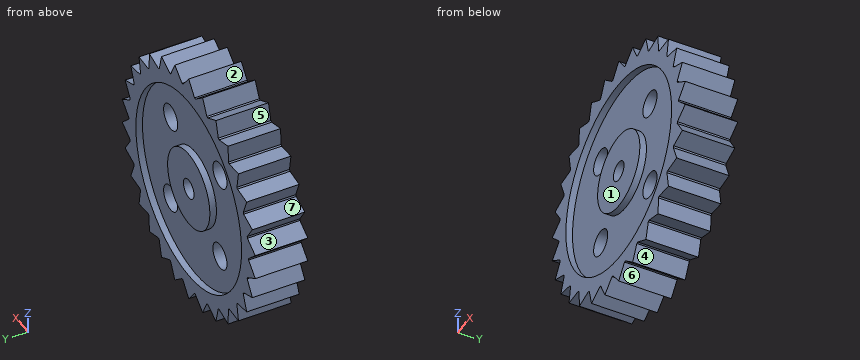
```python
from build123d import *

# Parameters (mm, degrees)
F0_R             = 13.49375
F1_DEPTH         = 3.175
F3_DEPTH         = 6.35
F3_COPIES_COUNT  = 30
F4_R             = 11.90625
F5_DEPTH         = 0.79375
F6_R             = 11.90625
F7_DEPTH         = 0.79375
F9_R             = 4.7625
F10_DEPTH        = 0.79375
F8_R             = 4.7625
F11_DEPTH        = 0.79375
F12_R            = 1.190625
F13_DEPTH        = 6.351
F14_R            = 1.5875
F15_DEPTH        = 5.55725
F15_COPIES_COUNT = 4


# Not quite as in the source:
# - a pattern or mirror of a feature is missing from the dataset's text; its kind, count and spacing are read off the source's solid


with BuildPart() as f1:
    # F0 (on Front) → F1 (new body, symmetric)
    with BuildSketch(Plane.XZ):
        Circle(F0_R)
    extrude(amount=F1_DEPTH, both=True)

    # F2 (on face) → F3 (join, through all)
    with BuildSketch(Plane.XZ.offset(3.175)):
        with BuildLine():
            Line((0, 15.08125), (-1.3182605719, 13.4292024382))
            ThreePointArc((-1.3182605719, 13.4292024382), (-0.6599199427, 13.4776034491), (0, 13.49375))
            Line((0, 13.49375), (0, 15.08125))
        make_face()
        with BuildLine():
            Line((1.2989129689, 13.4310876016), (0, 15.08125))
            Line((0, 15.08125), (0, 13.49375))
            ThreePointArc((0, 13.49375), (0.650211788, 13.4780752963), (1.2989129689, 13.4310876016))
        make_face()
    f3 = extrude(amount=-F3_DEPTH)

    # F3_copies: F3 ×30 about axis
    f3_copies_axis = Axis((0, 0, 0), (0, 1, 0))
    for i in range(1, F3_COPIES_COUNT):
        add(f3.rotate(f3_copies_axis, i * 360 / F3_COPIES_COUNT))

    # F4 (on face) → F5 (cut)
    with BuildSketch(Plane.XZ.offset(3.175)):
        Circle(F4_R)
    extrude(amount=-F5_DEPTH, mode=Mode.SUBTRACT)

    # F6 (on face) → F7 (cut)
    with BuildSketch(Plane(origin=(0, 3.175, 0), x_dir=(-1, 0, 0), z_dir=(0, 1, 0))):
        Circle(F6_R)
    extrude(amount=-F7_DEPTH, mode=Mode.SUBTRACT)

    # F9 (on face) → F10 (join)
    with BuildSketch(Plane(origin=(0, 2.38125, 0), x_dir=(-1, 0, 0), z_dir=(0, 1, 0))):
        Circle(F9_R)
    extrude(amount=F10_DEPTH)

    # F8 (on face) → F11 (join)
    with BuildSketch(Plane.XZ.offset(2.38125)):
        Circle(F8_R)
    extrude(amount=F11_DEPTH)

    # F12 (on face) → F13 (cut, through all)
    with BuildSketch(Plane.XZ.offset(3.175)):
        Circle(F12_R)
    extrude(amount=-F13_DEPTH, mode=Mode.SUBTRACT)

    # F14 (on face) → F15 (cut, through all)
    with BuildSketch(Plane.XZ.offset(2.38125)):
        with Locations((5.55625, -5.55625)):
            Circle(F14_R)
    f15 = extrude(amount=-F15_DEPTH, mode=Mode.SUBTRACT)

    # F15_copies: F15 ×4 about axis
    f15_copies_axis = Axis((0, 0, 0), (0, 1, 0))
    for i in range(1, F15_COPIES_COUNT):
        add(f15.rotate(f15_copies_axis, i * 360 / F15_COPIES_COUNT), mode=Mode.SUBTRACT)


solid = f1.part
```
Build history of the part. All positions in model axes, mm. Face numbers are marked on the shaded views. A direction names the side the tool comes from. Round coordinates to 2 decimals unless told otherwise and drop trailing zeros. Write each loop counter-clockwise with the first axis right and the second up, starting at its lowest first coordinate (ties: lowest second). Pieces come first, ordered by that corner, then holes.
1) Mould opens along X. For the marked faces 1, 2, 3 and 4 say: +X half, -X half, draft (parallel to the pull), parting line (faces both ways), or undercut.
2) Band-saw the part on A-A, the plane y = 2.75. Give the number of separate pieces and of enclosed holes in the cut face, and give its area (3 significant figures).
3) Band-saw the part on B-B, the plane z = -6. List the corners of the cut face in (x, y) (3 decimals).
4) Drill centre lines: probe 1 along X at (y, z) = (2.5, -3.5); probe 2 along X at (y, z) = (-1, -4.5); probe 3 along Y at (x, z) = (8.25, 7). Where is each one in solid material? Low to high.
5) 3-axis set-ups, long thin cutter, end or side, ignore diameter. For the marked faces 5, 6 and 7: which of +Z, -Z, +X, -X, +Y, -Y reach the whole face in a straight line?
6) Pin check, flat tips, straight feed: pin 1 (2 mm diameter, centred on x = -4, y = 1, fed in from -Z); pin 2 (1.5 mm diameter, centred on y = -2, z = 1.5, fed in from +X); pin 3 (6 mm diameter, centred on x = 3.5, z = -7.5, fed in from -Y). Stop position of each tip, or through.
Ans:
1. face 1: draft
1. face 2: undercut
1. face 3: -X half
1. face 4: undercut
2. separate pieces: 2
2. enclosed holes: 2
2. area: 255 mm2
3. outline: (-12.445, -3.175) - (-10.284, -3.175) - (-10.284, -2.381) - (-7.08, -2.381) - (-7.08, 2.381) - (-10.284, 2.381) - (-10.284, 3.175) - (-12.445, 3.175) - close; (-4.032, -2.381) - (4.032, -2.381) - (4.032, 2.381) - (-4.032, 2.381) - close; (7.08, -2.381) - (10.284, -2.381) - (10.284, -3.175) - (12.457, -3.175) - (12.457, 3.175) - (10.284, 3.175) - (10.284, 2.381) - (7.08, 2.381) - close
4. probe 1: x = -13.57 to -11.38, -3.23 to 3.23, 11.38 to 13.58
4. probe 2: x = -14.24 to -6.74, -4.37 to 4.37, 6.74 to 14.24
4. probe 3: y = -2.38 to 2.38
5. face 5: +Z, +Y, -Y
5. face 6: -Z, +Y, -Y
5. face 7: -X, +Y, -Y
6. pin 1: stops at z = -14.75
6. pin 2: stops at x = 15
6. pin 3: stops at y = -2.38
